Design review of the part built by this model. Coordinates are the model's own, in mm. A direction names the side the tool comes from. Give positions to 0.01 mm unless a question says otherwise; leave off trailing zeros. Loops run counter-clockwise (first coordinate to the right, second up) from the corner with the lowest first, then second, coordinate; pieces in that order, holes last. Notation, with made-up numbers: (-28.75, 24) - (-20.75, 24) arc R21 cw to (-20.75, 63) - close; hole circle Ø5 at (67.5, -34.5). An arc over 180 degrees is marked (long way). Write each question's results on one line, items separated by ' | '.
```python
from build123d import *


with BuildPart() as part:
    # Эскиз1 → Повернуть1 (revolve)
    with BuildSketch(Plane(origin=(0, 0, 0), x_dir=(1, 0, 0), z_dir=(0, 1, 0)), mode=Mode.PRIVATE) as revolve_1_sk:
        Polygon((-25, 0), (-17, 0), (-17, -115.6), (-20, -115.6), (-20, -100.6), (-25, -100.6), align=None)
    revolve_1 = revolve(revolve_1_sk.sketch.rotate(Axis((0, 0, 1000), (0, 0, -1)), 180), axis=Axis((0, 0, 1000), (0, 0, -1)))

    # Зеркальное отражение1: Повернуть1 across plane
    add(revolve_1.mirror(Plane(origin=(-25, 0, 0), x_dir=(1, 0, 0), z_dir=(0, 0, 1))))


solid = part.part
```
Item 1: We need section A-A on y = 0. Give the boundary of the cut face in (x, z), then the cut area to 3 significant figures.
Output values:
outline: (-25, -100.6) - (-20, -100.6) - (-20, -115.6) - (-17, -115.6) - (-17, 115.6) - (-20, 115.6) - (-20, 100.6) - (-25, 100.6) - close; (17, -115.6) - (20, -115.6) - (20, -100.6) - (25, -100.6) - (25, 100.6) - (20, 100.6) - (20, 115.6) - (17, 115.6) - close | area: 3,400 mm²
Item 2: Clearance check with flat-ended pins moving along their axes: P1, Ø1, axis at x = 11.5, z = 78.5, coming from the +Y side; P2, Ø6, axis at y = 19, z = -46.5, coming from the +X side; P3, Ø12, axis at x = -4.5, z = -46, coming from the +Y side. State where each tip first meets the part, or that it passes through.
Output values:
P1: stops at y = 22.45 | P2: stops at x = 19.21 | P3: stops at y = 25
Item 3: We need section C-C on z = -38. Give the boundary of the cut face in (x, y).
Output values:
outline: circle Ø50 at (0, 0); hole circle Ø34 at (0, 0)
Item 4: Draft analysis for pull direction Y (two halves, no side actions). For faces 3 (the face through (11, -17, -100.6)), 4 (the face through (-2.213, -16.855, -1.618)), 5 (the face through (-19.98, -0.88, -108)), state which applies: +Y half, -Y half, draft (parallel to the pull), parting line (faces both ways), or undercut.
Output values:
face 3: draft | face 4: undercut | face 5: parting line
Item 5: Tool access review of faces 1 (the face through (9, 15, 115.6)), 2 (the face through (11, -17, 100.6)): name each direction out of +Z, -Z, +X, -X, +Y, -Y from which nothing blocks a thin tool from reaching the whole face with its end or side.
Output values:
face 1: +Z, +X, -X, +Y, -Y | face 2: +Z
Item 6: Wall thickness on probe 1 along Y at (x, z) = (0, -68); probe 2 along Z at (x, y) = (-20, -14); probe 3 along X at (y, z) = (10, -46): over which ranges is each line inside the solid? List them lowest first.
Output values:
probe 1: y = -25 to -17, 17 to 25 | probe 2: z = -100.6 to 100.6 | probe 3: x = -22.91 to -13.75, 13.75 to 22.91
